```python
from build123d import *

# Parameters (mm, degrees)
SKETCH1_R           = 10.5
BOSS_EXTRUDE2_DEPTH = 27.94
SKETCH2_R           = 12.5
BOSS_EXTRUDE3_DEPTH = 2.54
SKETCH3_R           = 10
CUT_EXTRUDE2_DEPTH  = 25.4


with BuildPart() as part:
    # Sketch1 → Boss-Extrude2 (new body)
    with BuildSketch(Plane.XY):
        Circle(SKETCH1_R)
    extrude(amount=BOSS_EXTRUDE2_DEPTH)

    # Sketch2 → Boss-Extrude3 (add)
    with BuildSketch(Plane(origin=(0, 0, 0), x_dir=(-1, 0, 0), z_dir=(0, 0, -1))):
        Circle(SKETCH2_R)
    extrude(amount=-BOSS_EXTRUDE3_DEPTH)

    # Sketch3 → Cut-Extrude2 (cut)
    with BuildSketch(Plane(origin=(0, 0, 0), x_dir=(-1, 0, 0), z_dir=(0, 0, -1))):
        Circle(SKETCH3_R)
    extrude(amount=-CUT_EXTRUDE2_DEPTH, mode=Mode.SUBTRACT)


solid = part.part
```
Could you check a few things on this model? Use its own coordinates, in mm. A direction names the side the tool comes from. Coordinates: 2 decimals unless noted, no trailing zeros. Loops run counter-clockwise (first coordinate to the right, second up) from the corner with the lowest first, then second, coordinate; pieces in that order, holes last.
1) Will these pins go through, and if not, where does the flat tip stop? pin 1 Ø12 at (y, z) = (3, 5) entering from +X; pin 2 Ø1.5 at (y, z) = (-1, 16.5) entering from -X; pin 3 Ø12 at (y, z) = (-5.5, 16.5) entering from +X; pin 4 Ø6 at (x, y) = (-1, -3) entering from -Z.
Reported:
pin 1: stops at x = 12.5
pin 2: stops at x = -10.5
pin 3: stops at x = 10.5
pin 4: stops at z = 25.4
2) Please list where these lines run through material, in increasing order: line 1 along Y through (x, z) = (0, 10.25); line 2 along Z through (x, y) = (4.5, 7.5).
Reported:
line 1: y = -10.5 to -10, 10 to 10.5
line 2: z = 25.4 to 27.94
3) Which directions (+Z, -Z, +X, -X, +Y, -Y) give clear straight access to the entire face, cutting with the end or side of a thin tool? Please do faces 1 (the face through (0, 0, 27.94)), 2 (the face through (10, 3.2, 15.1)), 3 (the face through (2.17, -9.76, 12.52)).
Reported:
face 1: +Z, +X, -X, +Y, -Y
face 2: +Z
face 3: -Z
4) Thinking about a two-plate mould opening in Y: for faces 4 (the face through (0, 0, 25.4)), 5 (the face through (0.1, 10.2, 0)), 6 (the face through (-11.923, 3.755, 1.252)), which applies, released by +Y, released by -Y, zero draft, split by the parting line, or undercut?
Reported:
face 4: undercut
face 5: zero draft
face 6: split by the parting line
5) Imagine slicing it at D-D (z = 22.75). List the corners of the cut face in (x, y) for me.
Reported:
outline: circle Ø21 at (0, 0); hole circle Ø20 at (0, 0)
6) Imagine slicing it at B-B (z = 2). List the corners of the cut face in (x, y) for me, and give its area (3 significant figures).
Reported:
outline: circle Ø25 at (0, 0); hole circle Ø20 at (0, 0)
area: 177 mm2
7) Imagine slicing it at A-A (y = 0). List the corners of the cut face in (x, z) for me, and give its area (3 significant figures).
Reported:
outline: (-12.5, 0) - (-10, 0) - (-10, 25.4) - (10, 25.4) - (10, 0) - (12.5, 0) - (12.5, 2.54) - (10.5, 2.54) - (10.5, 27.94) - (-10.5, 27.94) - (-10.5, 2.54) - (-12.5, 2.54) - close
area: 88.9 mm2
